Geometry: see drawing. Coordinates: mm, zero at the bounding-box minimum. Round coordinates to 2 decimals unless told otherwise and drop trailing zeros. Loops run counter-clockwise (first coordinate to the right, second up) from the corner with the lowest first, then second, coordinate; pieces in that order, holes last. Notation, with made-up numbers: (39.5, 60.5) - (47.5, 60.5) arc R13 ccw to (47.5, 77.5) - close; hole circle Ø7 at (64.25, 87). An arc over 180 degrees is marked (long way). Use CSV: the item, a comma, the result in double quotes.
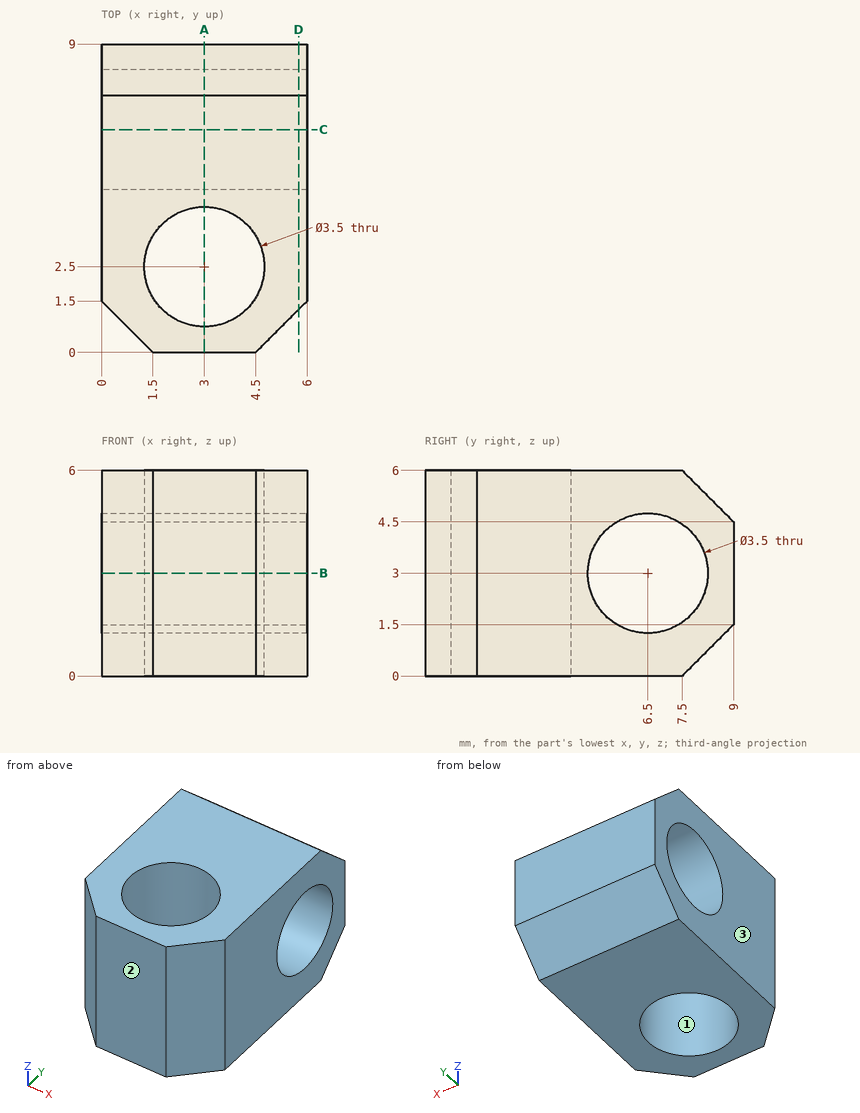
Item 1: Section A-A on x = 3. Return the cut outline in (y, z).
Final values:
outline,"(0, 0) - (0.75, 0) - (0.75, 6) - (0, 6) - close; (4.25, 0) - (7.5, 0) - (9, 1.5) - (9, 4.5) - (7.5, 6) - (4.25, 6) - close; hole circle Ø3.5 at (6.5, 3)"
Item 2: Material intervals for line 1 (X direction, y = 2.5, z = 4.5); line 2 (Y direction, x = 4, z = 3); line 3 (Y direction, x = 4.25, z = 3.5), sorted ascending.
Final values:
line 1,"x = 0 to 1.25, 4.75 to 6"
line 2,"y = 0 to 1.06, 3.94 to 4.75, 8.25 to 9"
line 3,"y = 0 to 1.28, 3.72 to 4.82, 8.18 to 9"
Item 3: Section B-B on z = 3. Return the cut outline in (x, y), plus the area to 3 significant figures.
Final values:
outline,"(0, 1.5) - (1.5, 0) - (4.5, 0) - (6, 1.5) - (6, 4.75) - (0, 4.75) - close; (0, 8.25) - (6, 8.25) - (6, 9) - (0, 9) - close; hole circle Ø3.5 at (3, 2.5)"
area,"21.1 mm²"
Item 4: Section D-D on x = 5.75. Return the cut outline in (y, z), plus the area to 3 significant figures.
Final values:
outline,"(1.25, 0) - (7.5, 0) - (9, 1.5) - (9, 4.5) - (7.5, 6) - (1.25, 6) - close; hole circle Ø3.5 at (6.5, 3)"
area,"34.6 mm²"
Item 5: Section C-C on y = 6.5. Return the cut outline in (x, z).
Final values:
outline,"(0, 0) - (6, 0) - (6, 1.25) - (0, 1.25) - close; (0, 4.75) - (6, 4.75) - (6, 6) - (0, 6) - close"
Item 6: Mould query, pull axis X, two halves, no side actions, for the marked faces 1, 2 and 3. Classes: released by +X, released by -X, zero draft, split by the parting line, or undercut.
Final values:
face 1,"undercut"
face 2,"zero draft"
face 3,"released by -X"
